The figure shows three views and two pictorial views of one solid part (mm, origin at its lowest corner). Answer the questions. A direction names the side the tool comes from. Coordinates: 2 decimals unless noted, no trailing zeros. Write each loop counter-clockwise with the first axis right and the second up, starting at its lowest first coordinate (ties: lowest second). Pieces come first, ordered by that corner, then holes. Notation, with made-up numbers: M 31,-16 L 79,-16 A28 ccw 79,13 Z; hole C 38,-34.75 d11. An arc over 180 degrees is marked long. Write item = value, one per line.
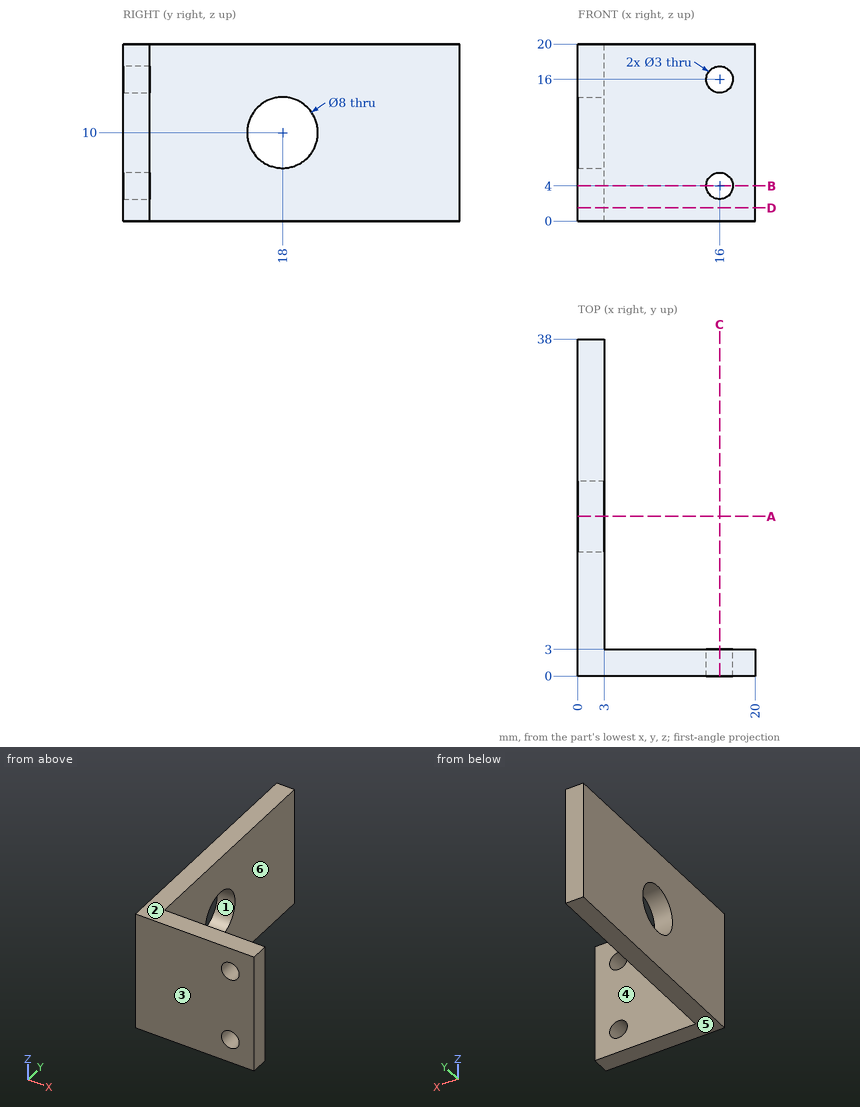
Item 1: Find section C-C (x = 16). Determine the outline of the cut face in (y, z), and give its area (3 significant figures).
Worked answers:
outline = M 0,0 L 3,0 L 3,2.5 L 0,2.5 Z; M 0,5.5 L 3,5.5 L 3,14.5 L 0,14.5 Z; M 0,17.5 L 3,17.5 L 3,20 L 0,20 Z
area = 42.0 mm²
Item 2: Consider line 1 along Z through (x, y) = (1.15, 18); line 2 along X through (y, z) = (1.25, 4); line 3 along Y through (x, z) = (7, 10.5). Determine where each line is inside the solid, lowest interval first. Write a range as from..to.
Worked answers:
line_1 = 0..6, 14..20
line_2 = 0..14.5, 17.5..20
line_3 = 0..3
Item 3: Find section B-B (z = 4). Determine the outline of the cut face in (x, y).
Worked answers:
outline = M 0,0 L 14.5,0 L 14.5,3 L 3,3 L 3,38 L 0,38 Z; M 17.5,0 L 20,0 L 20,3 L 17.5,3 Z
Item 4: Which of the six approach directions +Z, -Z, +X, -X, +Y, -Y give full straight-line access (tool end or side, diameter ignored) to the marked faces 5 and 6?
Worked answers:
face_5 = -Z, +X, -X, +Y, -Y
face_6 = +Z, -Z, +X, +Y
Item 5: Find section A-A (y = 18). Determine the outline of the cut face in (x, z), and give its area (3 significant figures).
Worked answers:
outline = M 0,0 L 3,0 L 3,6 L 0,6 Z; M 0,14 L 3,14 L 3,20 L 0,20 Z
area = 36.0 mm²
Item 6: For a pull along Y with two mould halves and no side action, classify the marked faces 1, 2, 3 and 4 as released by +Y, released by -Y, zero draft, split by the parting line, or undercut.
Worked answers:
face_1 = undercut
face_2 = zero draft
face_3 = released by -Y
face_4 = released by +Y
Item 7: Flat-ended cylindrical pins translate along their axes: pin 1 (12 mm diameter, centred on x = 14.5, z = 12.5, fed in from -Y); pin 2 (5 mm diameter, centred on y = 16, z = 6.5, fed in from +X); pin 3 (12 mm diameter, centred on x = 12, z = 3.5, fed in from +Y). Find the tip coordinate at first contact, or state that the pin passes through.
Worked answers:
pin_1 = 0
pin_2 = 3
pin_3 = 3
Item 8: Find section D-D (z = 1.5). Determine the outline of the cut face in (x, y).
Worked answers:
outline = M 0,0 L 20,0 L 20,3 L 3,3 L 3,38 L 0,38 Z
